CAD build for the part. Positions are in the model's coordinates, mm. A direction names the side the tool comes from. Round coordinates to 2 decimals unless told otherwise and drop trailing zeros. Loops run counter-clockwise (first coordinate to the right, second up) from the corner with the lowest first, then second, coordinate; pieces in that order, holes last. Notation, with made-up numbers: M 25,89 L 70,89 A6 ccw 70,93 Z; hole C 42,-15.5 d6. An arc over 180 degrees is marked long. Use a Markdown table: item, result. Add a question column.
(1) Band-saw the part on B-B, the plane y = 7. Write the cut outline in (x, z).
(2) Wall check: L1, parallel to X at y = 20, z = 30.5; L2, parallel to Y at x = 4, z = 4.5; L3, parallel to Y at x = 19, z = -1. Give the ranges that are in metal, low to high.
(3) Band-saw the part on C-C, the plane z = 8.5. Write the cut outline in (x, y), and give its area (3 significant figures).
(4) Two-plate mould, pull along Y, no slides. Class faces 6 (the face through (22, 26, 10.75)), 7 (the face through (22, 5, 6)), 8 (the face through (21.67, 33.5, -9.32)): released by +Y, released by -Y, zero draft, split by the parting line, or undercut.
(5) Flat gauge pins, fed straight in: P1, Ø7, axis at x = -23, y = 27, coming from the +Z side; P2, Ø7, axis at x = -20, z = 11, coming from the +Y side; P3, Ø11, axis at x = 2, z = 19, coming from the +Y side. Where does each tip first touch, or does it go through?
(6) Which spindle directions (+Z, -Z, +X, -X, +Y, -Y) get a long thin tool onto all of the face, cutting with end or side? Do faces 1 (the face through (-21.58, 33.57, -9.25)), 2 (the face through (0, 3, 12)), 3 (the face through (22, 23, 23)), 4 (the face through (22, 30.5, 0)), 5 (the face through (22, 35, 0)). Say none if no direction does.
(7) Band-saw the part on D-D, the plane x = 11. Write the cut outline in (y, z), and give its area (4 significant figures).
(8) Band-saw the part on A-A, the plane z = 3. Give the number of separate pieces and of enclosed holes in the cut face, and give its area (3 significant figures).
from build123d import *

# Parameters (mm, degrees)
SKETCH_1_W          = 49.5
SKETCH_1_H          = 21.5
EXTRUDE_1_DEPTH     = 3
SKETCH_4_W          = 6.25
SKETCH_4_H          = 21.5
EXTRUDE_2_DEPTH     = 20
EXTRUDE_3_DEPTH     = 25
SKETCH_7_W          = 6.25
SKETCH_7_H          = 21.5
EXTRUDE_4_DEPTH     = 12
SKETCH_8_W          = 8
SKETCH_8_H          = 5
CUT_EXTRUDE_1_DEPTH = 50.5
FILLET_1_R          = 5
FILLET_2_R          = 5
SKETCH_9_W          = 25
SKETCH_9_H          = 14
CUT_EXTRUDE_2_DEPTH = 50.5
CHAMFER_1_SIZE      = 1


with BuildPart() as part:
    # 草图1 → 凸台-拉伸1 (new body)
    with BuildSketch(Plane(origin=(0, 0, 0), x_dir=(1, 0, 0), z_dir=(0, 1, 0))):
        Rectangle(SKETCH_1_W, SKETCH_1_H)
    extrude(amount=EXTRUDE_1_DEPTH)

    # 草图4 → 凸台-拉伸2 (add)
    with BuildSketch(Plane(origin=(0, 3, 0), x_dir=(1, 0, 0), z_dir=(0, 1, 0))):
        with Locations((-21.625, 0)):
            Rectangle(SKETCH_4_W, SKETCH_4_H)
        with Locations((21.625, 0)):
            Rectangle(SKETCH_4_W, SKETCH_4_H)
    extrude(amount=EXTRUDE_2_DEPTH)

    # 草图6 → 凸台-拉伸3 (add)
    with BuildSketch(Plane.XY.offset(10.75)):
        Polygon((-24.75, 0), (24.75, 0), (24.75, 23), (18.5, 23), (18.5, 3), (-18.5, 3), (-18.5, 23), (-24.75, 23), align=None)
    extrude(amount=EXTRUDE_3_DEPTH)

    # 草图7 → 凸台-拉伸4 (add)
    with BuildSketch(Plane(origin=(0, 23, 0), x_dir=(1, 0, 0), z_dir=(0, 1, 0))):
        with Locations((-21.625, 0)):
            Rectangle(SKETCH_7_W, SKETCH_7_H)
        with Locations((21.625, 0)):
            Rectangle(SKETCH_7_W, SKETCH_7_H)
    extrude(amount=EXTRUDE_4_DEPTH)

    # 草图8 → 切除-拉伸1 (cut, through all)
    with BuildSketch(Plane(origin=(24.75, 0, 0), x_dir=(0, 0, -1), z_dir=(1, 0, 0))):
        with Locations((0, 28)):
            Rectangle(SKETCH_8_W, SKETCH_8_H)
    extrude(amount=-CUT_EXTRUDE_1_DEPTH, mode=Mode.SUBTRACT)

    # 圆角1
    fillet_1_edges = [part.edges().sort_by_distance(p)[0] for p in [
        (-21.625, 35, 10.75),
        (21.625, 35, 10.75),
    ]]
    fillet(fillet_1_edges, radius=FILLET_1_R)

    # 圆角2
    fillet_2_edges = [part.edges().sort_by_distance(p)[0] for p in [
        (-21.625, 35, -10.75),
        (21.625, 35, -10.75),
    ]]
    fillet(fillet_2_edges, radius=FILLET_2_R)

    # 草图9 → 切除-拉伸2 (cut, through all)
    with BuildSketch(Plane(origin=(24.75, 0, 0), x_dir=(0, 0, -1), z_dir=(1, 0, 0))):
        with Locations((-5.75, 12)):
            Rectangle(SKETCH_9_W, SKETCH_9_H)
    extrude(amount=-CUT_EXTRUDE_2_DEPTH, mode=Mode.SUBTRACT)

    # 倒角1
    chamfer_1_edges = [part.edges().sort_by_distance(p)[0] for p in [
        (18.5, 25.5, 0),
        (18.5, 28, -4),
        (18.5, 30.5, 0),
        (18.5, 28, 4),
        (-18.5, 28, 4),
        (-24.75, 28, 4),
        (-18.5, 30.5, 0),
        (-24.75, 30.5, 0),
        (-18.5, 28, -4),
        (-24.75, 28, -4),
        (-18.5, 25.5, 0),
        (-24.75, 25.5, 0),
        (24.75, 28, 4),
        (24.75, 25.5, 0),
        (24.75, 28, -4),
        (24.75, 30.5, 0),
    ]]
    chamfer(chamfer_1_edges, length=CHAMFER_1_SIZE)


solid = part.part
Return value:
| question | item | result |
|---|---|---|
| 1 | outline | M -24.75,-10.75 L -18.5,-10.75 L -18.5,-6.75 L -24.75,-6.75 Z; M -24.75,18.25 L -18.5,18.25 L -18.5,35.75 L -24.75,35.75 Z; M 18.5,-10.75 L 24.75,-10.75 L 24.75,-6.75 L 18.5,-6.75 Z; M 18.5,18.25 L 24.75,18.25 L 24.75,35.75 L 18.5,35.75 Z |
| 2 | L1 | -24.75 to -18.5, 18.5 to 24.75 |
| 2 | L2 | 0 to 3 |
| 2 | L3 | 0 to 5, 19 to 25, 31 to 35 |
| 3 | outline | M -24.75,0 L 24.75,0 L 24.75,5 L 18.5,5 L 18.5,3 L -18.5,3 L -18.5,5 L -24.75,5 Z; M -24.75,19 L -18.5,19 L -18.5,34.18 L -24.75,34.18 Z; M 18.5,19 L 24.75,19 L 24.75,34.18 L 18.5,34.18 Z |
| 3 | area | 363 mm^2 |
| 4 | face 6 | zero draft |
| 4 | face 7 | undercut |
| 4 | face 8 | released by +Y |
| 5 | P1 | z = 10.75 |
| 5 | P2 | y = 34.68 |
| 5 | P3 | y = 3 |
| 6 | face 1 | -Z, +X, -X, +Y |
| 6 | face 2 | +Z, -Z, +Y |
| 6 | face 3 | +Z, +X, -X, +Y |
| 6 | face 4 | +X, -X |
| 6 | face 5 | +Z, -Z, +X, -X, +Y |
| 7 | outline | M 0,-10.75 L 3,-10.75 L 3,35.75 L 0,35.75 Z |
| 7 | area | 139.5 mm^2 |
| 8 | separate pieces | 5 |
| 8 | enclosed holes | 0 |
| 8 | area | 307 mm^2 |
